Verification items for this drawing (mm, ordinates from the low corner). A direction names the side the tool comes from. Coordinates: 2 decimals unless noted, no trailing zeros. Write each loop counter-clockwise with the first axis right and the second up, starting at its lowest first coordinate (ties: lowest second). Pieces come first, ordered by that corner, then holes. Notation, with made-up numbers: M 58,4.25 L 86,4.25 A12 ccw 86,10.25 Z; hole C 48.25,84.25 d10. An arc over 180 degrees is marked long. Answer as CSV lines item,"result". Start each with the question number.
1) Section check C-C (z = 49). Record the cut outline in (x, y).
2) Section check A-A (y = 45.5). Record the cut outline in (x, z).
3) Go/stop test with flat-tipped pins: pin 1 Ø12.5 at (y, z) = (25, 49) entering from -X; pin 2 Ø24.5 at (x, z) = (54, 72.5) entering from -Y; pin 3 Ø5 at (x, z) = (93.5, 19) entering from +Y; pin 4 Ø12 at (x, y) = (78.5, 27) entering from -Z. Record where each tip stops, or that it passes through.
4) Section check B-B (x = 57). Record the cut outline in (y, z) (1 decimal), and give its area (3 significant figures).
5) Material ranges on L1, parallel to X at y = 14, z = 18.5; L2, parallel to Y at x = 44, z = 58; L3, parallel to Z at x = 99.5, y = 22, recorded low to high. Write a range as [from, to].
6) Access from +Z, -Z, +X, -X, +Y, -Y to the whole of each face (thin tool, end or side, straight path). Record for the marked faces 1, 2 and 3.
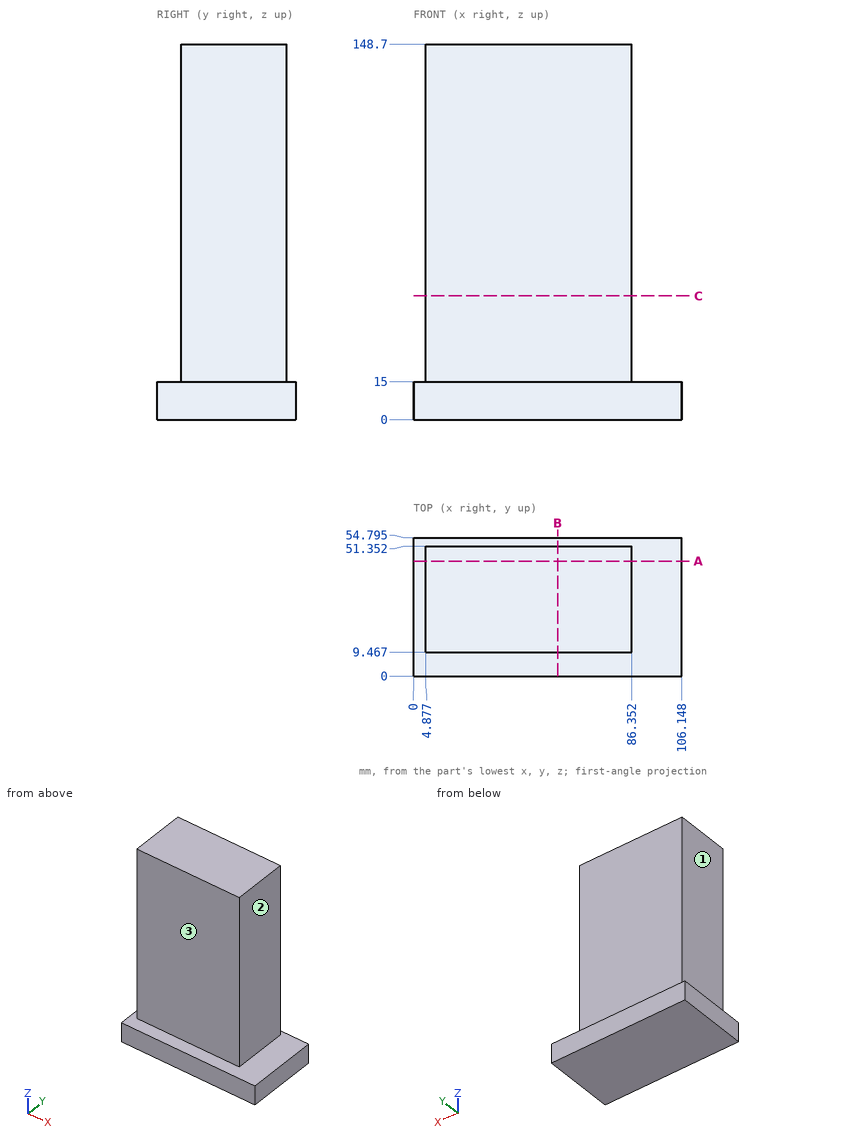
Results found:
1,outline,"M 4.88,9.47 L 86.35,9.47 L 86.35,51.35 L 4.88,51.35 Z"
2,outline,"M 0,0 L 106.15,0 L 106.15,15 L 86.35,15 L 86.35,148.7 L 4.88,148.7 L 4.88,15 L 0,15 Z"
3,pin 1,"stops at x = 4.88"
3,pin 2,"stops at y = 9.47"
3,pin 3,"passes through"
3,pin 4,"stops at z = 0"
4,outline,"M 0,0 L 54.8,0 L 54.8,15 L 51.4,15 L 51.4,148.7 L 9.5,148.7 L 9.5,15 L 0,15 Z"
4,area,"6,420 mm2"
5,L1,"x = [4.88, 86.35]"
5,L2,"y = [9.47, 51.35]"
5,L3,"z = [0, 15]"
6,face 1,"+Z, -X, +Y, -Y"
6,face 2,"+Z, +X, +Y, -Y"
6,face 3,"+Z, +X, -X, -Y"
